Check sheet for the modelled part. Datum: model origin and axes. Units: mm. A direction names the side the tool comes from. Coordinates: 2 decimals unless noted, no trailing zeros. Loops run counter-clockwise (first coordinate to the right, second up) from the corner with the lowest first, then second, coordinate; pieces in that order, holes last. Notation, with made-up numbers: (-10, -10.5) -> (48, -10.5) arc R17 cw to (48, -5.5) -> close; hole circle Ø8 at (74, 61). An arc over 180 degrees is marked (long way). Use CSV: the item, a comma, the result in double quotes. Start each with the question number.
1. Sectioned sample at C-C, the plane y = 0. Record the cut outline in (x, z), and give its area (3 significant figures).
2. Sectioned sample at A-A, the plane y = 10. Record the cut outline in (x, z), and give its area (3 significant figures).
3. Sectioned sample at D-D, the plane x = -3. Record the cut outline in (y, z).
4. Gauge pin test, flat ends, axial feed: pin 1 (9 mm diameter, centred on y = 0, z = 0, fed in from -X); pin 2 (3.5 mm diameter, centred on y = -5, z = -8.66, fed in from +X); pin 3 (1.3 mm diameter, centred on x = -3, y = -15, fed in from -Z). Record the tip position at first contact, or that the pin passes through.
5. Thickness scan on L1, parallel to Y at x = -3, z = -22.1; L2, parallel to Z at x = -0.3, y = -3; L3, parallel to Z at x = -0.6, y = 0. Record the ranges inside material, lowest first.
6. Set-up check for faces 1 (the face through (-3, -15, 20)), 2 (the face through (-2.512, 12.804, -22.535)), 3 (the face through (-1.972, -2.282, -7.804)), 4 (the face through (-2.96, -1.08, -4.88)): record each of +Z, -Z, +X, -X, +Y, -Y from which the full face is reachable in a straight line by a thin tool's end or side.
7. Sectioned sample at B-B, the plane z = 0. Record the cut outline in (x, y).
8. Release check for a two-part mould opening along Y. For faces 5 (the face through (-4.99, -5.35, 7.1)), 6 (the face through (-6, 0, 6)) record: pulls with the +Y half, pulls with the -Y half, needs draft (parallel to the pull), parting line crosses it, or undercut.
Autodesk Inventor part; units mm, degrees
ref_plane "YZ Plane" through (0, 0, 0) normal (1, 0, 0) x (0, 1, 0)
ref_plane "XZ Plane" through (0, 0, 0) normal (0, 1, 0) x (-1, 0, 0)
ref_plane "XY Plane" through (0, 0, 0) normal (0, 0, 1) x (1, 0, 0)
sketch "スケッチ1" plane through (0, 0, 0) normal (1, 0, 0) x (0, 1, 0)
  line L0 (-20, -25) -> (-20, 25)
  line L1 (-20, 25) -> (20, 25)
  line L2 (20, 25) -> (20, -25)
  line L3 (20, -25) -> (-20, -25)
  line L4 (-20, -25) -> (20, 25) construction
  line L5 (-20, 25) -> (20, -25) construction
  circle A0 centre (0, 0) radius 5
  circle A1 centre (10, 0) radius 1.6
  line L6 (0, 0) -> (18.1986, 0)
  circle A2 centre (10, 0) radius 2.85
  circle A3 centre (-5, 8.6603) radius 2.85
  circle A4 centre (-5, 8.6603) radius 1.6
  circle A5 centre (-5, -8.6603) radius 2.85
  circle A6 centre (-5, -8.6603) radius 1.6
  point P0 (0, 0)
  dimension "d0" = 40
  dimension "d1" = 50
  dimension "d8" = 10
  dimension "d9" = 10
  dimension "d10" = 3.2
  dimension "d11" = 5.7
  dimension "d14" = 360
extrude "押し出し1" add sketch "スケッチ1" against normal blind 6 contours L0 L1 L2 L3 | A0 | A2 L6 A1 | L6 A1 A2 | L6 A1 | A1 L6 | A3 | A4 | A5 | A6
extrude "押し出し2" cut sketch "スケッチ1" against normal blind 6 contours A0 | L6 A1 | A1 L6 | A4 | A6
extrude "押し出し3" cut sketch "スケッチ1" against normal blind 4 contours A2 L6 A1 | L6 A1 A2 | A3 | A5
sketch "スケッチ2" plane through (0, -20, 25) normal (0, 0, 1) x (1, 0, 0)
  circle A0 centre (-3, 5) radius 2.25
  circle A1 centre (-3, 35) radius 2.25
  line L0 (-6, 0) -> (-6, 40)
  line L1 (0, 0) -> (-6, 0)
  line L2 (0, 40) -> (-6, 40)
  point P0 (0, 20)
  dimension "d20" = 3
  dimension "d21" = 3
  dimension "d22" = 4.5
  dimension "d23" = 4.5
  dimension "d24" = 5
  dimension "d25" = 5
extrude "押し出し4" cut sketch "スケッチ2" against normal blind 5
sketch "スケッチ3" plane through (0, -20, -25) normal (0, 0, -1) x (-1, 0, 0)
  circle A0 centre (3, 5) radius 2.25
  circle A1 centre (3, 35) radius 2.25
  circle A2 centre (3, 5) radius 2.25
  circle A3 centre (3, 5) radius 2.25
  circle A4 centre (3, 35) radius 2.25
  point P0 (0, 20)
extrude "押し出し5" cut sketch "スケッチ3" against normal blind 5
properties part number "connect-wrist"
Completed:
1,outline,"(-6, -25) -> (0, -25) -> (0, -5) -> (-6, -5) -> close; (-6, 5) -> (0, 5) -> (0, 25) -> (-6, 25) -> close"
1,area,"240 mm²"
2,outline,"(-6, -25) -> (0, -25) -> (0, -2.85) -> (-4, -2.85) -> (-4, -1.6) -> (-6, -1.6) -> close; (-6, 1.6) -> (-4, 1.6) -> (-4, 2.85) -> (0, 2.85) -> (0, 25) -> (-6, 25) -> close"
2,area,"271 mm²"
3,outline,"(-20, -25) -> (-17.25, -25) -> (-17.25, -20) -> (-12.75, -20) -> (-12.75, -25) -> (12.75, -25) -> (12.75, -20) -> (17.25, -20) -> (17.25, -25) -> (20, -25) -> (20, 25) -> (17.25, 25) -> (17.25, 20) -> (12.75, 20) -> (12.75, 25) -> (-12.75, 25) -> (-12.75, 20) -> (-17.25, 20) -> (-17.25, 25) -> (-20, 25) -> close; hole circle Ø5.7 at (-5, -8.66); hole circle Ø5.7 at (-5, 8.66); hole circle Ø10 at (0, 0); hole circle Ø5.7 at (10, 0)"
4,pin 1,"through"
4,pin 2,"x = -4"
4,pin 3,"z = -20"
5,L1,"-20 to -17.25, -12.75 to 12.75, 17.25 to 20"
5,L2,"-25 to -10.69, -6.63 to -4, 4 to 6.63, 10.69 to 25"
5,L3,"-25 to -5, 5 to 25"
6,face 1,"+Z"
6,face 2,"-Z"
6,face 3,"+X"
6,face 4,"+X, -X"
7,outline,"(-6, -20) -> (0, -20) -> (0, -5) -> (-6, -5) -> close; (-6, 5) -> (0, 5) -> (0, 7.15) -> (-4, 7.15) -> (-4, 8.4) -> (-6, 8.4) -> close; (-6, 11.6) -> (-4, 11.6) -> (-4, 12.85) -> (0, 12.85) -> (0, 20) -> (-6, 20) -> close"
8,face 5,"undercut"
8,face 6,"needs draft"
